```python
from build123d import *

# Parameters (mm, degrees)
SKETCH1_R           = 10
BOSS_EXTRUDE1_DEPTH = 10


with BuildPart() as part:
    # Sketch1 → Boss-Extrude1 (new body)
    with BuildSketch(Plane.XY):
        with BuildLine():
            Line((-130, -20), (130, -20))
            ThreePointArc((130, -20), (150, 0), (130, 20))
            Line((130, 20), (-130, 20))
            ThreePointArc((-130, 20), (-150, 0), (-130, -20))
        make_face()
        with Locations((130, 0)):
            Circle(SKETCH1_R, mode=Mode.SUBTRACT)
        with Locations((-130, 0)):
            Circle(SKETCH1_R, mode=Mode.SUBTRACT)
        Polygon((-90, 10), (-85, 15), (85, 15), (-90, -10), align=None, mode=Mode.SUBTRACT)
        Polygon((-85, -15), (85, -15), (90, -10), (90, 10), align=None, mode=Mode.SUBTRACT)
    extrude(amount=BOSS_EXTRUDE1_DEPTH)


solid = part.part
```
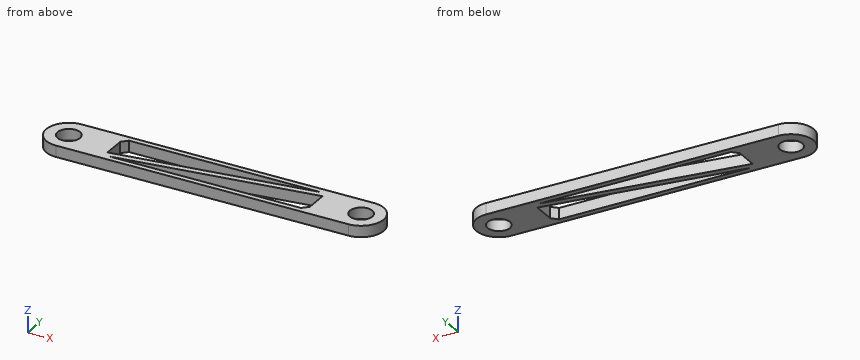
Geometry: final body of the model. Coordinates: model frame, mm. Give positions to 0.01 mm unless a question says otherwise; leave off trailing zeros. Order: outer loops, then holes, each group sorted by start corner. A loop starts at its lowest first (then second) coordinate and runs counter-clockwise, first axis right, second up. Notation, with made-up numbers: (84, -17.5) -> (98, -17.5) arc R13 ccw to (98, -3.5) -> close; hole circle Ø3 at (42.25, 17.5). An arc over 180 degrees is marked (long way). Write each question's results on one line, items separated by ' | '. Start each with the question number.
1) Section B-B (x = -67). Return loops of the section in (y, z).
2) Section C-C (z = 4.25). Return loops of the section in (x, y).
3) Section D-D (y = 12.5). Return loops of the section in (x, z), then the cut area to 3 significant figures.
4) Line query: line 1 (Y direction, x = -130, z = 6); line 2 (Y direction, x = 69, z = 2); line 3 (X direction, y = -15.5, z = 7). Output: solid intervals per line, ascending. Write a range as from..to.
5) Section A-A (y = 0). Return loops of the section in (x, z), then the cut area to 3 significant figures.
6) First-contact query: pin 1 (12 mm diameter, centred on x = 4.5, y = -3, fed in from -Z); pin 2 (3 mm diameter, centred on y = -3, z = 7, fed in from -X); pin 3 (5 mm diameter, centred on y = 0.5, z = 6.5, fed in from +X). Flat tips, straight axial feed; report the tip coordinate or a pass-through.
Calculated:
1) outline: (-20, 0) -> (-15, 0) -> (-15, 10) -> (-20, 10) -> close; (-12.43, 0) -> (-6.71, 0) -> (-6.71, 10) -> (-12.43, 10) -> close; (15, 0) -> (20, 0) -> (20, 10) -> (15, 10) -> close
2) outline: (-130, -20) -> (130, -20) arc R20 ccw to (130, 20) -> (-130, 20) arc R20 ccw to start; hole circle Ø20 at (-130, 0); hole (-90, -10) -> (85, 15) -> (-85, 15) -> (-90, 10) -> close; hole (-85, -15) -> (85, -15) -> (90, -10) -> (90, 10) -> close; hole circle Ø20 at (130, 0)
3) outline: (-145.61, 0) -> (-87.5, 0) -> (-87.5, 10) -> (-145.61, 10) -> close; (67.5, 0) -> (145.61, 0) -> (145.61, 10) -> (67.5, 10) -> close | area: 1,360 mm2
4) line 1: -20..-10, 10..20 | line 2: -20..-15, 7..12.71, 15..20 | line 3: -142.64..142.64
5) outline: (-150, 0) -> (-140, 0) -> (-140, 10) -> (-150, 10) -> close; (-120, 0) -> (-90, 0) -> (-90, 10) -> (-120, 10) -> close; (-20, 0) -> (20, 0) -> (20, 10) -> (-20, 10) -> close; (90, 0) -> (120, 0) -> (120, 10) -> (90, 10) -> close; (140, 0) -> (150, 0) -> (150, 10) -> (140, 10) -> close | area: 1,200 mm2
6) pin 1: z = 0 | pin 2: x = -149.94 | pin 3: x = 150
